from build123d import *

# Parameters (mm, degrees)
SKETCH1_W           = 55.88
SKETCH1_H           = 101.6
BOSS_EXTRUDE1_DEPTH = 2.54
SKETCH2_W           = 2.794
SKETCH2_H           = 31.326666666
SKETCH2_H_2         = 33.866666666
CUT_EXTRUDE1_DEPTH  = 59.032191067
SKETCH3_W           = 38.1
SKETCH3_H           = 81.28
CUT_EXTRUDE2_DEPTH  = 59.032191067
CAVITY1_START       = 48.26
CAVITY1_OUTLINE_W   = 18.499605322
CAVITY1_OUTLINE_H   = 2.54
CAVITY1_DEPTH       = 2.54


# Read off the part's stored shape, not the designer's step: Cavity1
with BuildPart() as part:
    # Sketch1 → Boss-Extrude1 (new body)
    with BuildSketch(Plane.XY):
        Rectangle(SKETCH1_W, SKETCH1_H)
    extrude(amount=BOSS_EXTRUDE1_DEPTH)

    # Sketch2 → Cut-Extrude1 (cut, through all)
    with BuildSketch(Plane(origin=(0, 0, 0), x_dir=(-1, 0, 0), z_dir=(0, 0, -1))):
        with Locations((-26.543, 0)):
            Rectangle(SKETCH2_W, SKETCH2_H)
        with Locations((26.543, 0)):
            Rectangle(SKETCH2_W, SKETCH2_H_2)
    extrude(amount=-CUT_EXTRUDE1_DEPTH, mode=Mode.SUBTRACT)

    # Sketch3 → Cut-Extrude2 (cut, through all)
    with BuildSketch(Plane.XY.offset(2.54)):
        Rectangle(SKETCH3_W, SKETCH3_H)
    extrude(amount=-CUT_EXTRUDE2_DEPTH, mode=Mode.SUBTRACT)

    # Cavity1 outline → Cavity1 (cut)
    with BuildSketch(Plane(origin=(0, 0, 0), x_dir=(1, 0, 0), z_dir=(0, 1, 0)).offset(CAVITY1_START)):
        with Locations((-0.190592016, -1.27)):
            Rectangle(CAVITY1_OUTLINE_W, CAVITY1_OUTLINE_H)
    extrude(amount=CAVITY1_DEPTH, mode=Mode.SUBTRACT)


solid = part.part
Work out the finished part from the listing and answer in its coordinate system (mm). A direction names the side the tool comes from. Round coordinates to 2 decimals unless told otherwise and drop trailing zeros. Write each loop counter-clockwise with the first axis right and the second up, starting at its lowest first coordinate (ties: lowest second). Pieces come first, ordered by that corner, then holes. Notation, with made-up numbers: (7.25, 17.25) - (64.25, 17.25) arc R6 cw to (64.25, 21.25) - close; hole circle Ø5 at (64.25, 68). An arc over 180 degrees is marked (long way). Answer in a Markdown table with one row per item. Add a question column.
1. A cutting plane is placed at A-A, the plane x = -16. Determine the outline of the cut face in (y, z).
2. A cutting plane is placed at C-C, the plane y = 28. Determine the outline of the cut face in (x, z).
3. Given pin 1 (1.3 mm diameter, centred on x = -2, z = 1, fed in from +Y); pin 2 (0.8 mm diameter, centred on y = 3.5, z = 1.5, fed in from +X); pin 3 (1.3 mm diameter, centred on y = 8.5, z = 1.5, fed in from -X), each flat-ended and moving along its own axis, determine where each tip first touches the part or whether it passes through.
4. The mould has two halves that part along X. Classify faces 1 (the flat face through (9.059, 50, 1)), 2 (the flat face through (-27.94, -34, 1)), 3 (the flat face through (-19, 50.8, 1)), 4 (the flat face through (27.94, 33, 1)): +X half, -X half, draft (parallel to the pull), parting line (faces both ways), or undercut.
5. For faces 5 (the flat face through (19.05, -1, 1)), 6 (the flat face through (-9.44, 50, 1)), 7 (the flat face through (25.146, 0, 1)), determine the directions among +Z, -Z, +X, -X, +Y, -Y from which every point of the face is accessible in a straight line to the end or side of a thin tool.
6. A cutting plane is placed at B-B, the plane z = 0.8. Determine the outline of the cut face in (x, y).
7. Find the intervals of material crossed by line 1 along Y through (x, z) = (11.5, 0.9); line 2 along X through (y, z) = (-15.5, 0.2); line 3 along Y through (x, z) = (5, 1.35), in increasing order. Write a range as from..to.
Worked out:
| question | item | result |
|---|---|---|
| 1 | outline | (-50.8, 0) - (-40.64, 0) - (-40.64, 2.54) - (-50.8, 2.54) - close; (40.64, 0) - (50.8, 0) - (50.8, 2.54) - (40.64, 2.54) - close |
| 2 | outline | (-27.94, 0) - (-19.05, 0) - (-19.05, 2.54) - (-27.94, 2.54) - close; (19.05, 0) - (27.94, 0) - (27.94, 2.54) - (19.05, 2.54) - close |
| 3 | pin 1 | y = 48.26 |
| 3 | pin 2 | x = 25.15 |
| 3 | pin 3 | x = -25.15 |
| 4 | face 1 | undercut |
| 4 | face 2 | -X half |
| 4 | face 3 | draft |
| 4 | face 4 | +X half |
| 5 | face 5 | +Z, -Z |
| 5 | face 6 | +Z, -Z, +Y |
| 5 | face 7 | +Z, -Z, +X |
| 6 | outline | (-27.94, -50.8) - (27.94, -50.8) - (27.94, -15.66) - (25.15, -15.66) - (25.15, 15.66) - (27.94, 15.66) - (27.94, 50.8) - (9.06, 50.8) - (9.06, 48.26) - (-9.44, 48.26) - (-9.44, 50.8) - (-27.94, 50.8) - (-27.94, 16.93) - (-25.15, 16.93) - (-25.15, -16.93) - (-27.94, -16.93) - close; hole (-19.05, -40.64) - (19.05, -40.64) - (19.05, 40.64) - (-19.05, 40.64) - close |
| 7 | line 1 | -50.8..-40.64, 40.64..50.8 |
| 7 | line 2 | -25.15..-19.05, 19.05..25.15 |
| 7 | line 3 | -50.8..-40.64, 40.64..48.26 |
